Input: dimensioned drawing with shaded views. Units: mm. Origin: part minimum x, y, z. A direction names the side the tool comes from. Coordinates: 2 decimals unless noted, no trailing zeros. Order: outer loops, then holes, each group sorted by start corner. A loop starts at its lowest first (then second) coordinate and runs counter-clockwise, first axis right, second up. Notation, with made-up numbers: (71.25, 33) -> (95.25, 33) arc R7 cw to (95.25, 40) -> close; hole circle Ø10 at (-38.5, 56.5). An arc over 180 degrees is marked (long way). Answer in a Markdown table with one row per item. Add a question column.
1) Contact query for flat-ended pins moving along their axis: P1, Ø5, axis at y = 24, z = 21.5, coming from the +X side (3 decimals); P2, Ø1, axis at y = 27, z = 15, coming from the -X side; P3, Ø2, axis at x = 3.5, z = 20, coming from the +Y side; P4, Ø1, axis at x = 1, z = 23, coming from the +Y side. Output: stop coordinate, or through.
2) Section query D-D on x = 2.5. Return the cut outline in (y, z), then the cut area to 3 significant figures.
3) Set-up query: the marked faces 1 and 2. Return all of +Z, -Z, +X, -X, +Y, -Y with unobstructed straight access to the full face (end or side cutting, diameter ignored); none if empty.
4) Section query A-A on z = 16. Count the separate pieces of the cut face and the enclosed holes in it, then the cut area to 3 significant figures.
5) Ray query, line 1 (Y direction, x = 2.25, z = 16); line 2 (X direction, y = 12, z = 10) (1 decimal); line 3 (Z direction, x = 3, y = 26) (1 decimal). Return the intervals inside material, ascending. Write a range as from..to.
6) Section query C-C on z = 5.5. Return the cut outline in (x, y) (1 decimal).
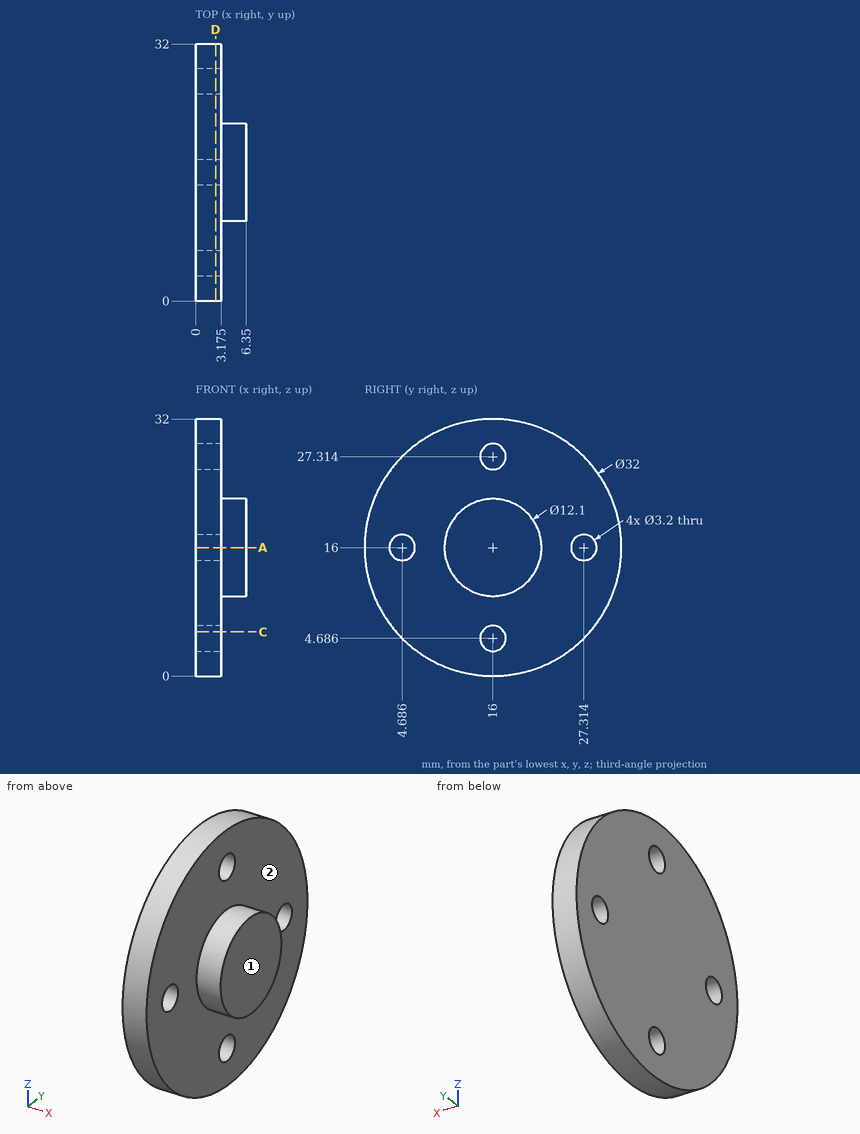
Result:
| question | item | result |
|---|---|---|
| 1 | P1 | x = 3.175 |
| 1 | P2 | through |
| 1 | P3 | y = 31.71 |
| 1 | P4 | y = 30.62 |
| 2 | outline | circle Ø32 at (16, 16); hole circle Ø3.2 at (4.69, 16); hole circle Ø3.2 at (16, 4.69); hole circle Ø3.2 at (16, 27.31); hole circle Ø3.2 at (27.31, 16) |
| 2 | area | 772 mm2 |
| 3 | face 1 | +Z, -Z, +X, +Y, -Y |
| 3 | face 2 | +X |
| 4 | separate pieces | 3 |
| 4 | enclosed holes | 0 |
| 4 | area | 120 mm2 |
| 5 | line 1 | 0..3.09, 6.29..25.71, 28.91..32 |
| 5 | line 2 | 0..3.2 |
| 5 | line 3 | 3.5..15.1, 16.9..28.5 |
| 6 | outline | (0, 3.9) -> (3.2, 3.9) -> (3.2, 14.6) -> (0, 14.6) -> close; (0, 17.4) -> (3.2, 17.4) -> (3.2, 28.1) -> (0, 28.1) -> close |
